```python
from build123d import *

# Parameters (mm, degrees)
SKETCH1_W                      = 160
SKETCH1_H                      = 1203
BOSS_EXTRUDE1_DEPTH            = 3.175
CONVERT_SOLID1_OUTLINE_W       = 160
CONVERT_SOLID1_OUTLINE_H       = 1203
CONVERT_SOLID1_DEPTH           = 0.13716
EDGE_FLANGE1_DEPTH             = 1203
EDGE_FLANGE2_START             = -160
EDGE_FLANGE2_DEPTH             = 160
EDGE_FLANGE2_2_DEPTH           = 923
EDGE_FLANGE3_DEPTH             = 923
EDGE_FLANGE3_BEND_DEPTH        = 160
F_9_5_9_5_DIAMETER_HOLE9_D     = 9.5
F_9_5_9_5_DIAMETER_HOLE9_DEPTH = 3.03784
F_9_5_9_5_DIAMETER_HOLE8_D     = 9.5
F_9_5_9_5_DIAMETER_HOLE8_DEPTH = 3.03784
M6_CLEARANCE_HOLE1_D           = 8.5
M8_CLEARANCE_HOLE1_D           = 9


# Read off the part's stored shape, not the designer's step: Convert-Solid1, Edge-Flange2
# Sheet-metal steps are written as plain solids
with BuildPart() as part:
    # Sketch1 → Boss-Extrude1 (new body)
    with BuildSketch(Plane(origin=(0, 0, 0), x_dir=(1, 0, 0), z_dir=(0, 1, 0))):
        with Locations((80, -601.5)):
            Rectangle(SKETCH1_W, SKETCH1_H)
    extrude(amount=BOSS_EXTRUDE1_DEPTH)

    # Convert-Solid1 outline → Convert-Solid1 (cut)
    with BuildSketch(Plane(origin=(0, 0, 0), x_dir=(1, 0, 0), z_dir=(0, 1, 0))):
        with Locations((80, -601.5)):
            Rectangle(CONVERT_SOLID1_OUTLINE_W, CONVERT_SOLID1_OUTLINE_H)
    extrude(amount=CONVERT_SOLID1_DEPTH, mode=Mode.SUBTRACT)

    # Edge-Flange1 section (across the edge) → Edge-Flange1 (add)
    with BuildSketch(Plane(origin=(163.175, 3.175, 1203), x_dir=(-1, 0, 0), z_dir=(0, 0, -1))):
        with BuildLine():
            Line((-3.03784, 3.175), (-3.03784, 26))
            Line((-3.03784, 26), (0, 26))
            Line((0, 26), (0, 3.175))
            ThreePointArc((0, 3.175), (0.92993597, 0.92993597), (3.175, 0))
            Line((3.175, 0), (3.175, -3.03784))
            ThreePointArc((3.175, -3.03784), (-1.218141294, -1.218141294), (-3.03784, 3.175))
        make_face()
    extrude(amount=EDGE_FLANGE1_DEPTH)

    # Edge-Flange2 outline → Edge-Flange2 (add)
    with BuildSketch(Plane(origin=(0, 3.175, 0), x_dir=(0, 0, 1), z_dir=(-1, 0, 0)).offset(EDGE_FLANGE2_START)):
        with BuildLine():
            Line((1209.21284, 58.74932), (1206.175, 58.74932))
            Line((1206.175, 58.74932), (1206.175, 3.175))
            ThreePointArc((1206.175, 3.175), (1205.24506403, 0.92993597), (1203, 0))
            Line((1203, 0), (1203, -3.03784))
            ThreePointArc((1203, -3.03784), (1207.393141294, -1.218141294), (1209.21284, 3.175))
            Line((1209.21284, 3.175), (1209.21284, 58.74932))
        make_face()
    extrude(amount=EDGE_FLANGE2_DEPTH)

    # Edge-Flange2 2 outline → Edge-Flange2 2 (add)
    with BuildSketch(Plane.XY):
        with BuildLine():
            Line((-6.21284, 61.92432), (-6.21284, 6.35))
            ThreePointArc((-6.21284, 6.35), (-4.393141294, 1.956858706), (0, 0.13716))
            Line((0, 0.13716), (0, 3.175))
            ThreePointArc((0, 3.175), (-2.24506403, 4.10493597), (-3.175, 6.35))
            Line((-3.175, 6.35), (-3.175, 61.92432))
            Line((-3.175, 61.92432), (-6.21284, 61.92432))
        make_face()
    extrude(amount=EDGE_FLANGE2_2_DEPTH)

    # Edge-Flange3 section (across the edge) → Edge-Flange3 (add)
    with BuildSketch(Plane(origin=(-3.175, 65.09932, 0), x_dir=(0, -1, 0), z_dir=(0, 0, 1))):
        with BuildLine():
            Line((-3.03784, 3.175), (-3.03784, 25))
            Line((-3.03784, 25), (0, 25))
            Line((0, 25), (0, 3.175))
            ThreePointArc((0, 3.175), (0.92993597, 0.92993597), (3.175, 0))
            Line((3.175, 0), (3.175, -3.03784))
            ThreePointArc((3.175, -3.03784), (-1.218141294, -1.218141294), (-3.03784, 3.175))
        make_face()
    extrude(amount=EDGE_FLANGE3_DEPTH)

    # Edge-Flange3 section 2 (across the edge) → Edge-Flange3 bend (add)
    with BuildSketch(Plane(origin=(0, 65.09932, 1206.175), x_dir=(0, -1, 0), z_dir=(1, 0, 0))):
        with BuildLine():
            Line((-3.03784, 3.175), (-3.03784, 25))
            Line((-3.03784, 25), (0, 25))
            Line((0, 25), (0, 3.175))
            ThreePointArc((0, 3.175), (0.92993597, 0.92993597), (3.175, 0))
            Line((3.175, 0), (3.175, -3.03784))
            ThreePointArc((3.175, -3.03784), (-1.218141294, -1.218141294), (-3.03784, 3.175))
        make_face()
    extrude(amount=EDGE_FLANGE3_BEND_DEPTH)

    # Ø9.5 (9.5) Diameter Hole9
    with Locations(Plane(origin=(166.21284, 0, 0), x_dir=(0, 0, -1), z_dir=(1, 0, 0))):
        with Locations((-98, 18.13716), (-458, 18.13716), (-818, 18.13716)):
            Hole(F_9_5_9_5_DIAMETER_HOLE9_D / 2, depth=F_9_5_9_5_DIAMETER_HOLE9_DEPTH)

    # Ø9.5 (9.5) Diameter Hole8
    with Locations(Plane(origin=(0, 68.13716, 0), x_dir=(1, 0, 0), z_dir=(0, 1, 0))):
        with Locations((11.21284, -98), (11.21284, -458), (11.21284, -818), (83.21284, -1198)):
            Hole(F_9_5_9_5_DIAMETER_HOLE8_D / 2, depth=F_9_5_9_5_DIAMETER_HOLE8_DEPTH)

    # M6 Clearance Hole1 (through all)
    with Locations(Plane(origin=(0, 3.175, 0), x_dir=(1, 0, 0), z_dir=(0, 1, 0))):
        with Locations((38.41286, -84.5878), (88.41286, -84.5878), (88.41286, -534.5878), (38.41286, -534.5878), (38.41286, -984.5878), (88.41286, -984.5878)):
            Hole(M6_CLEARANCE_HOLE1_D / 2)

    # M8 Clearance Hole1 (through all)
    with Locations(Plane(origin=(0, 0.13716, 0), x_dir=(-1, 0, 0), z_dir=(0, -1, 0))):
        with Locations((-19.05, -1152.06284), (-19.05, -1126.66284), (-19.05, -1101.26284), (-19.05, -1075.86284), (-19.05, -1050.46284)):
            Hole(M8_CLEARANCE_HOLE1_D / 2)


solid = part.part
```
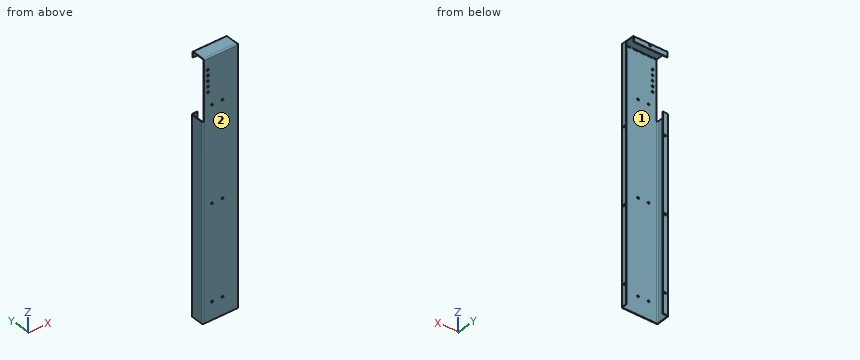
For this review, take the finished solid that the model builds, in its own axes (mm). Face numbers are marked on the shaded views. Give positions to 0.01 mm unless a question says otherwise; leave off trailing zeros. Write each loop counter-clockwise with the first axis right and the second up, starting at its lowest first coordinate (ties: lowest second). Pieces come first, ordered by that corner, then holes. Notation, with made-up numbers: M 62.25,-5.75 L 76.25,-5.75 A30 ccw 76.25,16.25 Z; hole C 83.5,-3.75 d9. An arc over 180 degrees is marked long. One line per item, written item: value.
1) The part is to be moulded in two halves that separate along X. For the marked faces 1 and 2, say which applies: +X half, -X half, draft (parallel to the pull), parting line (faces both ways), or undercut.
Results are:
face 1: undercut
face 2: draft
2) Take a section at A-A, the plane y = 39. Write out the cut boundary in (x, z) (3 decimals), then the cut area to 3 significant figures.
Results are:
outline: M -6.213,0 L -3.175,0 L -3.175,923 L -6.213,923 Z; M 0,1206.175 L 160,1206.175 L 160,1209.213 L 0,1209.213 Z
area: 3,290 mm²
3) For P1, Ø12, axis at y = 38.5, z = 135, coming from the +X side (3 decimals); P2, Ø3, axis at x = 72.5, y = 8.5, coming from the -Z side (3 decimals); P3, Ø12, axis at x = 32, z = 584.5, coming from the +Y side (3 decimals), all flat-tipped, find the tip position at first contact; note any pin that passes through.
Results are:
P1: stops at x = -3.175
P2: stops at z = 1206.175
P3: stops at y = 3.175
4) Take a section at B-B, the plane z = 408. Write out the cut boundary in (x, y) (3 decimals), then the cut area to 3 significant figures.
Results are:
outline: M -6.213,6.35 A6.213 ccw 0,0.137 L 160,0.137 A6.213 ccw 166.213,6.35 L 166.213,29.175 L 163.175,29.175 L 163.175,6.35 A3.175 cw 160,3.175 L 0,3.175 A3.175 cw -3.175,6.35 L -3.175,61.924 A3.175 cw 0,65.099 L 21.825,65.099 L 21.825,68.137 L 0,68.137 A6.213 ccw -6.213,61.924 Z
area: 858 mm²
5) For line 1 (Z direction, x = 19, y = 1); line 2 (X direction, y = 23, z = 631) (3 decimals); line 3 (Y direction, x = 4, z = 408) (3 decimals), list the stretches that pass through material, from the lowest coordinate up. Write a range as from..to.
Results are:
line 1: z = 0..1045.96, 1054.96..1071.36, 1080.36..1096.76, 1105.76..1122.16, 1131.16..1147.56, 1156.56..1206.16
line 2: x = -6.213..-3.175, 163.175..166.213
line 3: y = 0.137..3.175, 65.099..68.137
